Read the model definition and answer for the solid it produces. Units are mm, in the model's axes. Face numbers are marked on the shaded views. A direction names the side the tool comes from. Give positions to 0.01 mm unless a question says otherwise; leave off trailing zeros. Put each result on its own line as item: value. Start each with the question number.
1. For the marked faces 5 and 6, determine the directions among +Z, -Z, +X, -X, +Y, -Y from which every point of the face is accessible in a straight line to the end or side of a thin tool.
2. For a pull along X with two mould halves and no side action, classify the marked faces 1, 2, 3 and 4 as released by +X, released by -X, zero draft, split by the parting line, or undercut.
3. Given pin 1 Ø10 at (x, z) = (3.5, 7.5) entering from -Y; pin 2 Ø8 at (y, z) = (2, 10.5) entering from -X; pin 3 Ø5 at (x, y) = (6.5, -9.5) entering from -Z; pin 4 Ø6 at (x, z) = (-7, 10) entering from +Y, each flat-ended and moving along its own axis, determine where each tip first touches the part or whether it passes through.
4. Consider L1, parallel to X at y = 6.5, z = 1.5 (3 decimals); L2, parallel to Y at x = 0.5, z = 16.25. Determine where each line is inside the solid, lowest interval first. Write a range as from..to.
```python
from build123d import *

# Parameters (mm, degrees)
F0_W     = 30.48
F0_H     = 30.48
F0_W_2   = 26.67
F0_H_2   = 26.67
F1_DEPTH = 2.286
F2_DEPTH = 3.81


with BuildPart() as f1:
    # F0 (on Top) → F1 (new body)
    with BuildSketch(Plane.XY):
        Rectangle(F0_W, F0_H)
        Rectangle(F0_W_2, F0_H_2, mode=Mode.SUBTRACT)
    extrude(amount=-F1_DEPTH)

    # F0 (on Top) → F2 (join)
    with BuildSketch(Plane.XY):
        Rectangle(F0_W, F0_H)
        Rectangle(F0_W_2, F0_H_2, mode=Mode.SUBTRACT)
    extrude(amount=F2_DEPTH)

    # F5 (on face) → F6 section 0
    with BuildSketch(Plane.XY.offset(3.81)):
        Polygon((-13.335, 13.335), (-15.24, 15.24), (-15.24, -15.24), (-13.335, -13.335), align=None)
    # F4 (on offset) → F6 section 1
    with BuildSketch(Plane.XY.offset(16.51)):
        Polygon((-6.35, -4.445), (-6.35, 8.255), (-8.255, 10.16), (-8.255, -6.35), align=None)
    loft()

    # F5 (on face) → F7 section 0
    with BuildSketch(Plane.XY.offset(3.81)):
        Polygon((-15.24, -15.24), (15.24, -15.24), (13.335, -13.335), (-13.335, -13.335), align=None)
    # F4 (on offset) → F7 section 1
    with BuildSketch(Plane.XY.offset(16.51)):
        Polygon((8.255, -6.35), (6.35, -4.445), (-6.35, -4.445), (-8.255, -6.35), align=None)
    loft()

    # F5 (on face) → F8 section 0
    with BuildSketch(Plane.XY.offset(3.81)):
        Polygon((15.24, -15.24), (15.24, 15.24), (13.335, 13.335), (13.335, -13.335), align=None)
    # F4 (on offset) → F8 section 1
    with BuildSketch(Plane.XY.offset(16.51)):
        Polygon((8.255, 10.16), (6.35, 8.255), (6.35, -4.445), (8.255, -6.35), align=None)
    loft()

    # F5 (on face) → F9 section 0
    with BuildSketch(Plane.XY.offset(3.81)):
        Polygon((13.335, 13.335), (15.24, 15.24), (-15.24, 15.24), (-13.335, 13.335), align=None)
    # F4 (on offset) → F9 section 1
    with BuildSketch(Plane.XY.offset(16.51)):
        Polygon((-6.35, 8.255), (6.35, 8.255), (8.255, 10.16), (-8.255, 10.16), align=None)
    loft()


solid = f1.part
```
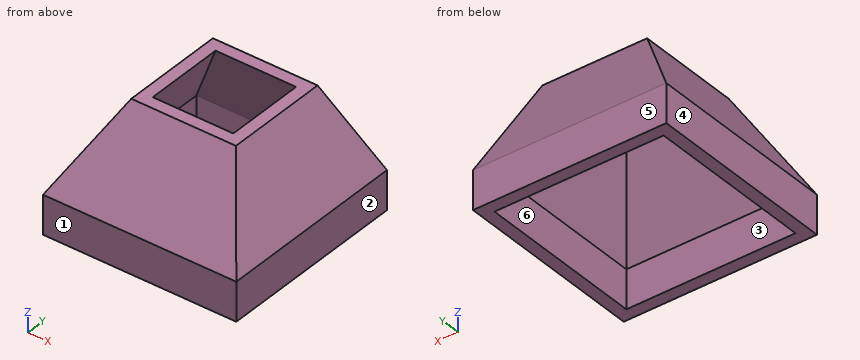
Return value:
1. face 5: +Z, -Z, +X, -X, +Y
1. face 6: -Z
2. face 1: zero draft
2. face 2: released by +X
2. face 3: undercut
2. face 4: released by -X
3. pin 1: stops at y = -15.24
3. pin 2: stops at x = -13.76
3. pin 3: stops at z = 5.72
3. pin 4: stops at y = 13.96
4. L1: x = -15.24..-13.335, 13.335..15.24
4. L2: y = -6.53..-4.63, 8.36..10.26
